```python
from build123d import *

# Parameters (mm, degrees)
BOSS_EXTRUDE1_DEPTH = 8
SKETCH2_R           = 2.75
CUT_EXTRUDE1_DEPTH  = 9
SKETCH3_R           = 5
CUT_EXTRUDE2_DEPTH  = 4.2
M5_TAPPED_HOLE1_D   = 4.2


with BuildPart() as part:
    # Sketch1 → Boss-Extrude1 (new body)
    with BuildSketch(Plane(origin=(0, 0, 0), x_dir=(1, 0, 0), z_dir=(0, 1, 0))):
        Polygon((7.5, 25), (6.5, 25), (6.5, -25), (7.5, -25), (7.5, -35), (-7.5, -35), (-7.5, 35), (7.5, 35), align=None)
    extrude(amount=BOSS_EXTRUDE1_DEPTH)

    # Sketch2 → Cut-Extrude1 (cut, through all)
    with BuildSketch(Plane(origin=(0, 8, 0), x_dir=(1, 0, 0), z_dir=(0, 1, 0))):
        with Locations((-0.5, 17.5)):
            Circle(SKETCH2_R)
        with Locations((-0.5, -17.5)):
            Circle(SKETCH2_R)
    extrude(amount=-CUT_EXTRUDE1_DEPTH, mode=Mode.SUBTRACT)

    # Sketch3 → Cut-Extrude2 (cut)
    with BuildSketch(Plane(origin=(0, 8, 0), x_dir=(1, 0, 0), z_dir=(0, 1, 0))):
        with Locations((-0.5, 17.5)):
            Circle(SKETCH3_R)
        with Locations((-0.5, -17.5)):
            Circle(SKETCH3_R)
    extrude(amount=-CUT_EXTRUDE2_DEPTH, mode=Mode.SUBTRACT)

    # M5 Tapped Hole1 (through all)
    with Locations(Plane(origin=(0, 8, 0), x_dir=(1, 0, 0), z_dir=(0, 1, 0))):
        with Locations((-0.5, 6.5)):
            Hole(M5_TAPPED_HOLE1_D / 2)


solid = part.part
```
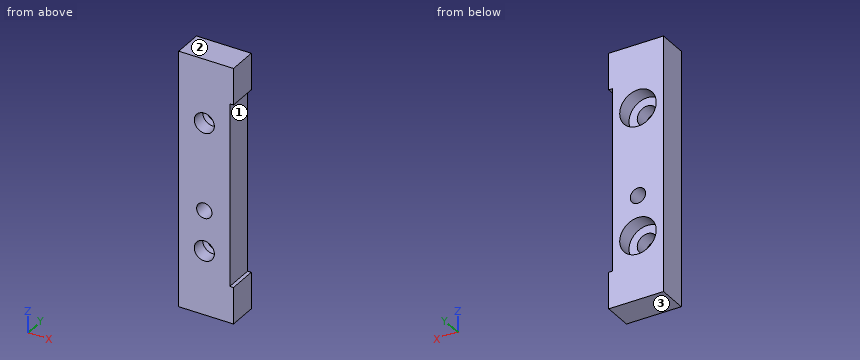
Read the model definition and answer for the solid it produces. Units are mm, in the model's axes. Face numbers are marked on the shaded views. Coordinates: 2 decimals unless noted, no trailing zeros. Loops run counter-clockwise (first coordinate to the right, second up) from the corner with the lowest first, then second, coordinate; pieces in that order, holes last.
(1) Flat-ended cylindrical pins translate along their axes: pin 1 Ø2 at (x, z) = (2.5, -9.5) entering from -Y; pin 2 Ø1 at (y, z) = (6, 21.5) entering from +X; pin 3 Ø7 at (x, z) = (-0.5, 17.5) entering from +Y. Find the tip coordinate at first contact, or state that the pin passes through.
Solution:
pin 1: stops at y = 0
pin 2: stops at x = 6.5
pin 3: stops at y = 3.8
(2) The part is cut by section D-D (z = -6.5). Determine the outline of the cut face in (x, y), and give its area (3 significant figures).
Solution:
outline: (-7.5, 0) - (-2.6, 0) - (-2.6, 8) - (-7.5, 8) - close; (1.6, 0) - (6.5, 0) - (6.5, 8) - (1.6, 8) - close
area: 78.4 mm2
(3) The part is cut by section A-A (z = 17.5). Determine the outline of the cut face in (x, y), and give its area (3 significant figures).
Solution:
outline: (-7.5, 0) - (-3.25, 0) - (-3.25, 3.8) - (-5.5, 3.8) - (-5.5, 8) - (-7.5, 8) - close; (2.25, 0) - (6.5, 0) - (6.5, 8) - (4.5, 8) - (4.5, 3.8) - (2.25, 3.8) - close
area: 49.1 mm2
(4) The part is cut by section B-B (y = 6.75). Determine the outline of the cut face in (x, z).
Solution:
outline: (-7.5, -35) - (7.5, -35) - (7.5, -25) - (6.5, -25) - (6.5, 25) - (7.5, 25) - (7.5, 35) - (-7.5, 35) - close; hole circle Ø10 at (-0.5, -17.5); hole circle Ø10 at (-0.5, 17.5); hole circle Ø4.2 at (-0.5, -6.5)
(5) The part is cut by section C-C (x = 0.75). Determine the outline of the cut face in (y, z).
Solution:
outline: (0, -35) - (8, -35) - (8, -22.34) - (3.8, -22.34) - (3.8, -19.95) - (0, -19.95) - close; (0, -15.05) - (3.8, -15.05) - (3.8, -12.66) - (8, -12.66) - (8, -8.19) - (0, -8.19) - close; (0, -4.81) - (8, -4.81) - (8, 12.66) - (3.8, 12.66) - (3.8, 15.05) - (0, 15.05) - close; (0, 19.95) - (3.8, 19.95) - (3.8, 22.34) - (8, 22.34) - (8, 35) - (0, 35) - close
(6) The mould has two halves that part along Z. Classify the marked faces 1, 2 and 3: released by +Z, released by -Z, zero draft, split by the parting line, or undercut.
Solution:
face 1: undercut
face 2: released by +Z
face 3: released by -Z
(7) Consider line 1 along Z through (x, y) = (-0.5, 4); line 2 along Z through (x, y) = (-0.25, 0.5); line 3 along Z through (x, y) = (-4.5, 7). Determine where each line is inside the solid, lowest interval first.
Solution:
line 1: z = -35 to -22.5, -12.5 to -8.6, -4.4 to 12.5, 22.5 to 35
line 2: z = -35 to -20.24, -14.76 to -8.59, -4.41 to 14.76, 20.24 to 35
line 3: z = -35 to -20.5, -14.5 to 14.5, 20.5 to 35
